Geometry check sheet. Reference: the model listing, model coordinates, mm. A direction names the side the tool comes from. Coordinates: 2 decimals unless noted, no trailing zeros. Loops run counter-clockwise (first coordinate to the right, second up) from the corner with the lowest first, then second, coordinate; pieces in that order, holes last.
from build123d import *

# Parameters (mm, degrees)
SKETCH1_W           = 41.91
SKETCH1_H           = 36.068
BOSS_EXTRUDE1_DEPTH = 12.7
SKETCH3_W           = 21.844
SKETCH3_H           = 27.94
CUT_EXTRUDE1_DEPTH  = 13.7
SKETCH4_W           = 16.002
SKETCH4_H           = 36.068
CUT_EXTRUDE2_DEPTH  = 6.35
SKETCH5_W           = 12.446
SKETCH5_H           = 22.86
CUT_EXTRUDE3_DEPTH  = 7.35
SKETCH6_R           = 1.016
SKETCH6_W           = 3.556
SKETCH6_H           = 2.54
CUT_EXTRUDE11_DEPTH = 6.35
CUT_EXTRUDE13_DEPTH = 1.524
SKETCH9_R           = 3.302
CUT_EXTRUDE14_DEPTH = 37.068


with BuildPart() as part:
    # Sketch1 → Boss-Extrude1 (new body)
    with BuildSketch(Plane(origin=(0, 0, 0), x_dir=(1, 0, 0), z_dir=(0, 1, 0))):
        Rectangle(SKETCH1_W, SKETCH1_H)
    extrude(amount=BOSS_EXTRUDE1_DEPTH)

    # Sketch3 → Cut-Extrude1 (cut, through all)
    with BuildSketch(Plane(origin=(0, 12.7, 0), x_dir=(1, 0, 0), z_dir=(0, 1, 0))):
        with Locations((10.033, 0)):
            Rectangle(SKETCH3_W, SKETCH3_H)
    extrude(amount=-CUT_EXTRUDE1_DEPTH, mode=Mode.SUBTRACT)

    # Sketch4 → Cut-Extrude2 (cut)
    with BuildSketch(Plane(origin=(0, 12.7, 0), x_dir=(1, 0, 0), z_dir=(0, 1, 0))):
        with Locations((-12.954, 0)):
            Rectangle(SKETCH4_W, SKETCH4_H)
    extrude(amount=-CUT_EXTRUDE2_DEPTH, mode=Mode.SUBTRACT)

    # Sketch5 → Cut-Extrude3 (cut, through all)
    with BuildSketch(Plane(origin=(0, 6.35, 0), x_dir=(1, 0, 0), z_dir=(0, 1, 0))):
        with Locations((-12.954, 0)):
            Rectangle(SKETCH5_W, SKETCH5_H)
    extrude(amount=-CUT_EXTRUDE3_DEPTH, mode=Mode.SUBTRACT)

    # Sketch6 → Cut-Extrude11 (cut)
    with BuildSketch(Plane(origin=(0, 6.35, 0), x_dir=(1, 0, 0), z_dir=(0, 1, 0))):
        with Locations((-12.954, -13.462)):
            Circle(SKETCH6_R)
        with Locations((-12.954, 13.462)):
            Circle(SKETCH6_R)
        with Locations((-12.954, -11.43)):
            Rectangle(SKETCH6_W, SKETCH6_H)
        with Locations((-12.954, 11.43)):
            Rectangle(SKETCH6_W, SKETCH6_H)
    extrude(amount=-CUT_EXTRUDE11_DEPTH, mode=Mode.SUBTRACT)

    # Sketch8 → Cut-Extrude13 (cut)
    with BuildSketch(Plane(origin=(0, 0, -18.034), x_dir=(-1, 0, 0), z_dir=(0, 0, -1))):
        with BuildLine():
            ThreePointArc((-1.143, 4.172598162), (1.034401838, 6.35), (-1.143, 8.527401838))
            Line((-1.143, 8.527401838), (-15.113, 9.652))
            ThreePointArc((-15.113, 9.652), (-18.415, 6.35), (-15.113, 3.048))
            Line((-15.113, 3.048), (-1.143, 4.172598162))
        make_face()
    cut_extrude13 = extrude(amount=-CUT_EXTRUDE13_DEPTH, mode=Mode.SUBTRACT)

    # Mirror1: Cut-Extrude13 across plane
    add(cut_extrude13.mirror(Plane.XY), mode=Mode.SUBTRACT)

    # Sketch9 → Cut-Extrude14 (cut, through all)
    with BuildSketch(Plane(origin=(0, 0, -18.034), x_dir=(-1, 0, 0), z_dir=(0, 0, -1))):
        with Locations((-15.113, 6.35)):
            Circle(SKETCH9_R)
    extrude(amount=-CUT_EXTRUDE14_DEPTH, mode=Mode.SUBTRACT)


solid = part.part
(1) Scan lines: L1, parallel to X at y = 2, z = 0 (3 decimals); L2, parallel to X at y = 6.5, z = 17 (3 decimals); L3, parallel to Z at x = -7.5, y = 5. Record each from-to range of solid material in increasing order.
Findings:
L1: x = -20.955 to -19.177, -6.731 to -0.889
L2: x = -4.953 to -1.029, 18.412 to 20.955
L3: z = -18.03 to -11.43, 11.43 to 18.03
(2) Sectioned sample at B-B on z = -6.5. Record the cut outline in (x, y) (3 decimals).
Findings:
outline: (-20.955, 0) - (-19.177, 0) - (-19.177, 6.35) - (-20.955, 6.35) - close; (-6.731, 0) - (-0.889, 0) - (-0.889, 12.7) - (-4.953, 12.7) - (-4.953, 6.35) - (-6.731, 6.35) - close
(3) Gauge pin test, flat ends, axial feed: pin 1 Ø1 at (x, y) = (-0.5, 7.5) entering from -Z; pin 2 Ø3 at (y, z) = (8, 7) entering from +X; pin 3 Ø1.9 at (y, z) = (8, 3) entering from -X. Record the tip position at first contact, or that the pin passes through.
Findings:
pin 1: stops at z = -18.03
pin 2: stops at x = -0.89
pin 3: stops at x = -4.95
(4) Access from +Z, -Z, +X, -X, +Y, -Y to the whole of each face (thin tool, end or side, straight path). Record for faces 1 (the flat face through (-11.176, 3, 12)), 2 (the flat face through (20.955, 6, -16)), 3 (the flat face through (7, 6, -16.51)), 4 (the flat face through (10, 6, -13.97)), 5 (the flat face through (-4.953, 10, 0)).
Findings:
face 1: +Y, -Y
face 2: +Z, -Z, +X, +Y, -Y
face 3: -Z
face 4: +X, +Y, -Y
face 5: +Z, -Z, -X, +Y
(5) Sectioned sample at A-A on x = -8. Record the cut outline in (y, z), and give its area (3 significant figures).
Findings:
outline: (0, -18.03) - (6.35, -18.03) - (6.35, -11.43) - (0, -11.43) - close; (0, 11.43) - (6.35, 11.43) - (6.35, 18.03) - (0, 18.03) - close
area: 83.9 mm2
(6) Sectioned sample at C-C on y = 2. Record the cut outline in (x, z) (3 decimals).
Findings:
outline: (-20.955, -18.034) - (20.955, -18.034) - (20.955, -13.97) - (-0.889, -13.97) - (-0.889, 13.97) - (20.955, 13.97) - (20.955, 18.034) - (-20.955, 18.034) - close; hole (-19.177, -11.43) - (-14.732, -11.43) - (-14.732, -12.7) - (-13.626, -12.7) arc R1.016 ccw (long way) to (-12.282, -12.7) - (-11.176, -12.7) - (-11.176, -11.43) - (-6.731, -11.43) - (-6.731, 11.43) - (-11.176, 11.43) - (-11.176, 12.7) - (-12.282, 12.7) arc R1.016 ccw (long way) to (-13.626, 12.7) - (-14.732, 12.7) - (-14.732, 11.43) - (-19.177, 11.43) - close
(7) Sectioned sample at D-D on y = 7.25. Record the cut outline in (x, z) (3 decimals), and give its area (3 significant figures).
Findings:
outline: (-4.953, -18.034) - (-0.84, -18.034) - (-0.84, -16.51) - (11.936, -16.51) - (11.936, -13.97) - (-0.889, -13.97) - (-0.889, 13.97) - (11.936, 13.97) - (11.936, 16.51) - (-0.84, 16.51) - (-0.84, 18.034) - (-4.953, 18.034) - close; (18.29, -18.034) - (20.955, -18.034) - (20.955, -13.97) - (18.29, -13.97) - close; (18.29, 13.97) - (20.955, 13.97) - (20.955, 18.034) - (18.29, 18.034) - close
area: 234 mm2
(8) Draft check along Y on faces 6 (the flat face through (-0.889, 6, 0)), 7 (the cylindrical face through (18.41, 6.5, 15.52)). Enter one of: +Y half, -Y half, draft (parallel to the pull), parting line (faces both ways), or undercut.
Findings:
face 6: draft
face 7: undercut
